Could you check a few things on this model? Use its own coordinates, in mm. Face numbers are marked on the shaded views. A direction names the side the tool comes from. Give positions to 0.01 mm unless a question says otherwise; leave off trailing zeros. Write each loop counter-clockwise with the first axis right and the second up, starting at its lowest first coordinate (ties: lowest second). Pieces come first, ordered by that corner, then holes. Notation, with made-up numbers: (-23.75, -10) - (18.25, -10) arc R30 ccw to (18.25, 27) - close; hole circle Ø5 at (14, -17.75). An arc over 180 degrees is marked (long way). Answer in a Markdown table with one row per item.
from build123d import *

# Parameters (mm, degrees)
F0_W      = 8.636
F0_H      = 9.652
F1_DEPTH  = 41.275
F2_R      = 2.54
F3_DEPTH  = 25.4
F5_R      = 1.651
F6_DEPTH  = 8.636
F7_R      = 4.7625
F8_DEPTH  = 0.889
F9_R      = 4.7625
F10_DEPTH = 0.889
F4_W      = 12.710963
F4_H      = 3.461967
F11_DEPTH = 9.652


with BuildPart() as f1:
    # F0 (on Right) → F1 (new body)
    with BuildSketch(Plane.YZ):
        Rectangle(F0_W, F0_H)
    extrude(amount=F1_DEPTH)

    # F2 (on face) → F3 (cut)
    with BuildSketch(Plane.YZ.offset(41.275)):
        Circle(F2_R)
    extrude(amount=-F3_DEPTH, mode=Mode.SUBTRACT)

    # F5 (on face) → F6 (cut)
    with BuildSketch(Plane.XZ.offset(4.318)):
        with Locations((5.08, 0)):
            Circle(F5_R)
    extrude(amount=-F6_DEPTH, mode=Mode.SUBTRACT)

    # F7 (on face) → F8 (cut)
    with BuildSketch(Plane.XZ.offset(4.318)):
        with Locations((5.08, 0)):
            Circle(F7_R)
    extrude(amount=-F8_DEPTH, mode=Mode.SUBTRACT)

    # F9 (on face) → F10 (cut)
    with BuildSketch(Plane(origin=(0, 4.318, 0), x_dir=(-1, 0, 0), z_dir=(0, 1, 0))):
        with Locations((-5.08, 0)):
            Circle(F9_R)
    extrude(amount=-F10_DEPTH, mode=Mode.SUBTRACT)

    # F4 (on face) → F11 (cut)
    with BuildSketch(Plane.XY.offset(4.826)):
        with Locations((6.355481, 0.034316)):
            Rectangle(F4_W, F4_H)
    extrude(amount=-F11_DEPTH, mode=Mode.SUBTRACT)


solid = f1.part
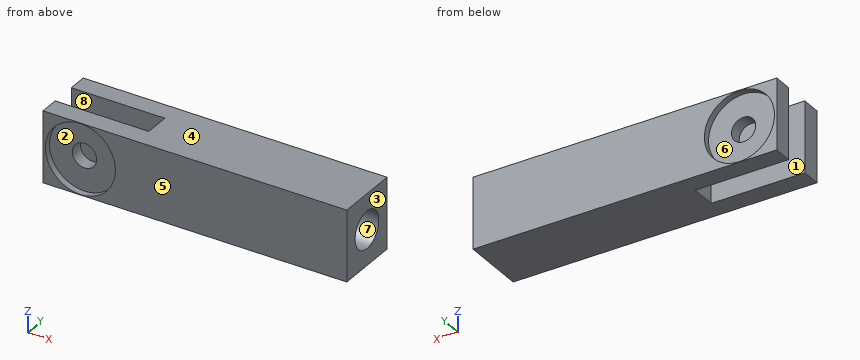
1) Imagine slicing it at B-B (z = 0). State how many separate pieces and enclosed holes the cut face has, then the cut area to 3 significant figures.
Check values:
| item | result |
|---|---|
| separate pieces | 3 |
| enclosed holes | 0 |
| area | 155 mm2 |
2) Imagine slicing it at A-A (x = 5.08). List the corners of the cut face in (y, z) for me.
Check values:
| item | result |
|---|---|
| outline | (-4.32, -4.83) - (-1.7, -4.83) - (-1.7, -1.65) - (-3.43, -1.65) - (-3.43, -4.76) - (-4.32, -4.76) - close; (-4.32, 4.76) - (-3.43, 4.76) - (-3.43, 1.65) - (-1.7, 1.65) - (-1.7, 4.83) - (-4.32, 4.83) - close; (1.77, -4.83) - (4.32, -4.83) - (4.32, -4.76) - (3.43, -4.76) - (3.43, -1.65) - (1.77, -1.65) - close; (1.77, 1.65) - (3.43, 1.65) - (3.43, 4.76) - (4.32, 4.76) - (4.32, 4.83) - (1.77, 4.83) - close |
3) If I drill on line 1 (Y direction, x = 2.5, z = -0.75); line 2 (Z direction, x = 26.25, y = 0); line 3 (Z direction, x = 5.08, y = 2.6), over which ranges is the centre line in solid material (lowest first)?
Check values:
| item | result |
|---|---|
| line 1 | y = -3.43 to -1.7, 1.77 to 3.43 |
| line 2 | z = -4.83 to -2.54, 2.54 to 4.83 |
| line 3 | z = -4.83 to -1.65, 1.65 to 4.83 |
4) Will these pins go through, and if not, where does the flat tip stop? P1, Ø5, axis at x = 5.5, z = 1.5, coming from the -Y side; P2, Ø5, axis at x = 4.5, z = 1.5, coming from the +Y side; P3, Ø1, axis at y = 0.5, z = -1, coming from the -X side; P4, Ø2.5, axis at x = 5.08, z = 0, coming from the +Y side.
Check values:
| item | result |
|---|---|
| P1 | stops at y = -3.43 |
| P2 | stops at y = 3.43 |
| P3 | stops at x = 12.71 |
| P4 | passes through |
5) We'd pull the mould along X, two halves only. Please class the marked faces 1, 2 and 3: +X half, -X half, draft (parallel to the pull), parting line (faces both ways), or undercut.
Check values:
| item | result |
|---|---|
| face 1 | draft |
| face 2 | undercut |
| face 3 | +X half |
6) Imagine slicing it at D-D (x = 29.5). List the corners of the cut face in (y, z) for me, then the cut area to 3 significant figures.
Check values:
| item | result |
|---|---|
| outline | (-4.32, -4.83) - (4.32, -4.83) - (4.32, 4.83) - (-4.32, 4.83) - close; hole circle Ø5.08 at (0, 0) |
| area | 63.1 mm2 |
7) Imagine slicing it at C-C (y = 0). List the corners of the cut face in (x, z) for me (3 decimals), then the cut area to 3 significant figures.
Check values:
| item | result |
|---|---|
| outline | (12.711, -4.826) - (41.275, -4.826) - (41.275, -2.54) - (15.875, -2.54) - (15.875, 2.54) - (41.275, 2.54) - (41.275, 4.826) - (12.711, 4.826) - close |
| area | 147 mm2 |
8) On a 3-axis mill with a long thin cutter (end or side, diameter ignored), from which of +Z, -Z, +X, -X, +Y, -Y can I reach the whole of each face in a straight line? I mean the marked faces 4, 5, 6, 7 and 8. Say none if no direction works.
Check values:
| item | result |
|---|---|
| face 4 | +Z, +X, -X, +Y, -Y |
| face 5 | +Z, -Z, +X, -X, -Y |
| face 6 | +Y |
| face 7 | +X |
| face 8 | +Z, -Z, -X |
